Can you work these out from the drawing? Everything is in mm from the part's minimum corner. A direction names the side the tool comes from. Coordinates: 2 decimals unless noted, no trailing zeros. Order: outer loops, then holes, each group sorted by start corner. A loop starts at its lowest first (then second) coordinate and runs counter-clockwise, first axis right, second up. Notation, with made-up numbers: (82.5, 64.25) -> (126.5, 64.25) arc R11 ccw to (126.5, 79.25) -> close; hole circle Ø4 at (58, -28.5). An arc over 180 degrees is marked (long way). Return JSON: item names as keys, results as strings. Group by question number.
1) If we section it at D-D, the plane y = 19.5: Please give me the cut outline in (x, z).
2) If I drill on probe 1 along Z at (x, y) = (33, 15.5); probe 2 along Z at (x, y) = (18.5, 21); probe 3 along Y at (x, z) = (13, 240), over which ranges is the centre line in solid material (lowest first)? Write a range as from..to.
3) If we section it at C-C, the plane x = 23: Please give me the cut outline in (y, z), then the cut area to 3 significant figures.
4) If we section it at A-A, the plane x = 5: Please give me the cut outline in (y, z), then the cut area to 3 significant figures.
5) For the marked faces 1, 2, 3, 4 and 5, which set-ups out of +Z, -Z, +X, -X, +Y, -Y let a thin tool reach every point of the face, with its end or its side?
6) If we section it at B-B, the plane z = 30.5: Please give me the cut outline in (x, y).
7) For pin 1 (4 mm diameter, centred on x = 23, z = 158, fed in from +Y); pin 2 (10 mm diameter, centred on y = 18.5, z = 136.5, fed in from -X); pin 3 (22 mm diameter, centred on x = 16.5, z = 145, fed in from -Y), each with a flat end and sliding along its axis, tell me the tip position at first contact or that it passes through.
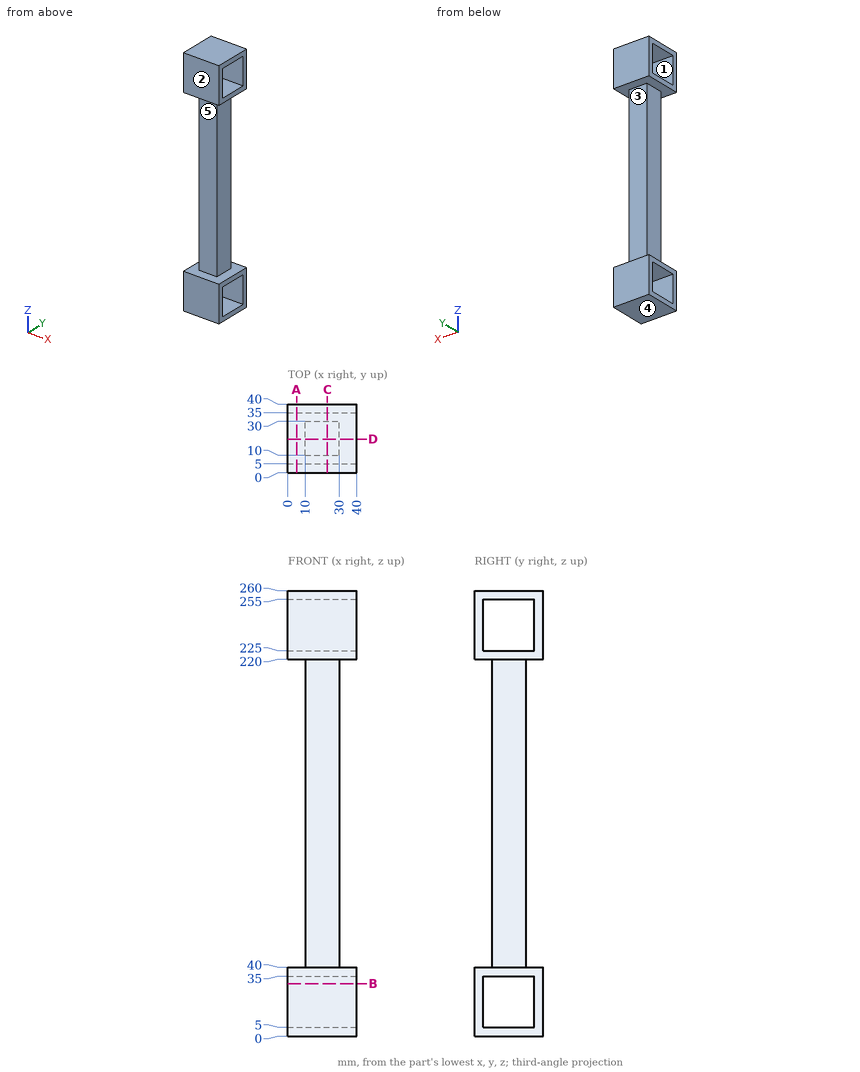
Result sheet:
{
 "1": {"outline": "(0, 0) -> (40, 0) -> (40, 5) -> (0, 5) -> close; (0, 35) -> (40, 35) -> (40, 40) -> (30, 40) -> (30, 220) -> (40, 220) -> (40, 225) -> (0, 225) -> (0, 220) -> (10, 220) -> (10, 40) -> (0, 40) -> close; (0, 255) -> (40, 255) -> (40, 260) -> (0, 260) -> close"},
 "2": {"probe 1": "z = 0..5, 35..40, 220..225, 255..260", "probe 2": "z = 0..5, 35..225, 255..260", "probe 3": "y = 0..5, 35..40"},
 "3": {"outline": "(0, 0) -> (40, 0) -> (40, 40) -> (30, 40) -> (30, 220) -> (40, 220) -> (40, 260) -> (0, 260) -> (0, 220) -> (10, 220) -> (10, 40) -> (0, 40) -> close; hole (5, 5) -> (35, 5) -> (35, 35) -> (5, 35) -> close; hole (5, 225) -> (35, 225) -> (35, 255) -> (5, 255) -> close", "area": "5,000 mm2"},
 "4": {"outline": "(0, 0) -> (40, 0) -> (40, 40) -> (0, 40) -> close; (0, 220) -> (40, 220) -> (40, 260) -> (0, 260) -> close; hole (5, 5) -> (35, 5) -> (35, 35) -> (5, 35) -> close; hole (5, 225) -> (35, 225) -> (35, 255) -> (5, 255) -> close", "area": "1,400 mm2"},
 "5": {"face 1": "+X, -X", "face 2": "+Z, -Z, +X, -X, -Y", "face 3": "+X, -X, +Y", "face 4": "-Z, +X, -X, +Y, -Y", "face 5": "+X, -X, -Y"},
 "6": {"outline": "(0, 0) -> (40, 0) -> (40, 5) -> (0, 5) -> close; (0, 35) -> (40, 35) -> (40, 40) -> (0, 40) -> close"},
 "7": {"pin 1": "stops at y = 30", "pin 2": "stops at x = 10", "pin 3": "stops at y = 10"}
}
